Source: CAD feature listing. Evaluate the final solid. Frame: model axes, mm. Face numbers are marked on the shaded views. A direction names the side the tool comes from. Coordinates: 2 decimals unless noted, no trailing zeros. Write item = value, one per line. Start each with the question number.
Item 1: Contact query for flat-ended pins moving along their axis: pin 1 (16.5 mm diameter, centred on x = -16.5, y = 26.5, fed in from +Z) (3 decimals); pin 2 (1 mm diameter, centred on y = -9.5, z = 29, fed in from +X); pin 3 (1 mm diameter, centred on x = 59.5, y = 12.5, fed in from +Z). Output: stop coordinate, or through.
Item 2: Ray query, line 1 along Z through (x, y) = (-21, -39.5) (3 decimals); line 2 along Y through (x, z) = (-1, 22); line 3 along Y through (x, z) = (33, 45). Return the intervals inside material, ascending. Write a range as [from, to].
Item 3: Set-up query: the marked faces 1, 2, 3, 4 and 5. Return all of +Z, -Z, +X, -X, +Y, -Y with unobstructed straight access to the full face (end or side cutting, diameter ignored); none if empty.
Item 4: Mould query, pull axis X, two halves, no side actions, for the marked faces 6, 7 and 8. Classes: released by +X, released by -X, zero draft, split by the parting line, or undercut.
```python
from build123d import *

# Parameters (mm, degrees)
F1_DEPTH = 63.5
F0_W     = 25.4
F0_H     = 19.05
F0_H_2   = 4.7498
F0_H_3   = 4.7752
F2_DEPTH = 25.4
F3_DEPTH = 7.9375
F5_R     = 5.08


with BuildPart() as f1:
    # F0 (on Front) → F1 (new body, symmetric)
    with BuildSketch(Plane.XZ):
        Polygon((22.225, 9.525), (-41.275, 9.525), (-41.275, -9.525), (41.275, -9.525), (41.275, 9.525), align=None)
    extrude(amount=F1_DEPTH, both=True)

    # F0 (on Front) → F2 (join, symmetric)
    with BuildSketch(Plane.XZ):
        with BuildLine():
            Line((22.225, 27.0002), (22.225, 9.525))
            Line((22.225, 9.525), (41.275, 9.525))
            Line((41.275, 9.525), (41.275, 27.0002))
            ThreePointArc((41.275, 27.0002), (45.9246798487, 38.2255201513), (57.15, 42.8752))
            Line((57.15, 42.8752), (60.325, 42.8752))
            Line((60.325, 42.8752), (60.325, 61.9252))
            Line((60.325, 61.9252), (57.15, 61.9252))
            ThreePointArc((57.15, 61.9252), (54.6822905468, 61.8379099571), (52.2269164674, 61.5764761663))
            ThreePointArc((52.2269164674, 61.5764761663), (30.77108496, 49.8892468633), (22.225, 27.0002))
        make_face()
        with Locations((73.025, 52.4002)):
            Rectangle(F0_W, F0_H)
        with Locations((73.025, 64.3001)):
            Rectangle(F0_W, F0_H_2)
        with Locations((73.025, 40.4876)):
            Rectangle(F0_W, F0_H_3)
    extrude(amount=F2_DEPTH, both=True)

    # F0 (on Front) → F3 (join, symmetric)
    with BuildSketch(Plane.XZ):
        with BuildLine():
            add(Edge.make_bspline(
                [(-41.275, 9.525), (-14.7710740566, 59.7766935825), (28.1573608518, 65.3158426285), (52.2269164674, 61.5764761663)],
                knots=[0, 0, 0, 0, 107.0138521602, 107.0138521602, 107.0138521602, 107.0138521602], degree=3))
            Line((-41.275, 9.525), (22.225, 9.525))
            Line((22.225, 9.525), (22.225, 27.0002))
            ThreePointArc((22.225, 27.0002), (30.77108496, 49.8892468633), (52.2269164674, 61.5764761663))
        make_face()
    extrude(amount=F3_DEPTH, both=True)

    # F0 (on Front) → F4 (revolve)
    with BuildSketch(Plane.XZ):
        Polygon((85.725, 66.675), (85.725, 61.9252), (85.725, 42.8752), (85.725, 38.1), (111.125, 38.1), (111.125, 66.675), align=None)
    revolve(axis=Axis((85.725, 0, 52.3875), (0, 0, 1)))

    # F5
    f5_edges = [f1.edges().sort_by_distance(p)[0] for p in [
        (41.275, 63.5, 0),
        (41.275, -63.5, 0),
        (-41.275, -63.5, 0),
        (-41.275, 63.5, 0),
    ]]
    fillet(f5_edges, radius=F5_R)


solid = f1.part
```
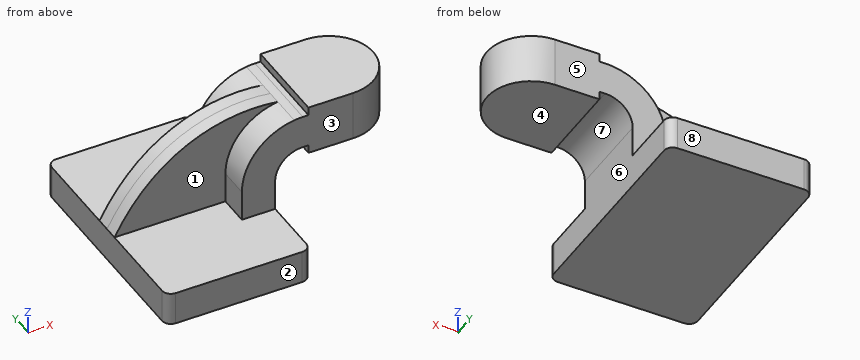
Computed:
q1.pin_1 = 9.525
q1.pin_2 = 41.47
q1.pin_3 = 61.93
q2.line_1 = [-9.525, 9.525]
q2.line_2 = [-7.94, 7.94]
q2.line_3 = [-25.4, 25.4]
q3.face_1 = +Z, -X, -Y
q3.face_2 = +Z, -Z, +X, -X, -Y
q3.face_3 = +Z, +X, -X, -Y
q3.face_4 = -Z, +X, +Y, -Y
q3.face_5 = +Z, +X, -X, +Y
q4.face_6 = released by +X
q4.face_7 = undercut
q4.face_8 = zero draft
